Read the model definition and answer for the solid it produces. Units are mm, in the model's axes. A direction names the side the tool comes from. Coordinates: 2 decimals unless noted, no trailing zeros. Loops run counter-clockwise (first coordinate to the right, second up) from the corner with the lowest first, then second, coordinate; pieces in that order, holes last.
from build123d import *

# Parameters (mm, degrees)
F0_W      = 304.8
F0_H      = 304.8
F1_DEPTH  = 38.1
F2_W      = 228.6
F2_H      = 228.6
F3_DEPTH  = 38.1
F4_W      = 38.1
F4_H      = 38.1
F5_DEPTH  = 1143
F6_W      = 304.8
F6_H      = 304.8
F7_DEPTH  = 38.1
F8_W      = 228.6
F8_H      = 228.6
F9_DEPTH  = 38.1
F10_W     = 38.1
F10_H     = 38.1
F11_DEPTH = 342.9
F12_W     = 38.1
F12_H     = 38.1
F13_DEPTH = 342.9
F14_R     = 6.35
F16_DEPTH = 0.254
F15_R     = 6.35
F17_DEPTH = 0.254
F18_W     = 38.1
F18_H     = 38.1
F19_DEPTH = 304.8


with BuildPart() as f1:
    # F0 (on Top) → F1 (new body)
    with BuildSketch(Plane.XY):
        Rectangle(F0_W, F0_H)
    extrude(amount=-F1_DEPTH)

    # F2 (on face) → F3 (cut)
    with BuildSketch(Plane.XY):
        Rectangle(F2_W, F2_H)
    extrude(amount=-F3_DEPTH, mode=Mode.SUBTRACT)

    # F4 (on face) → F5 (join)
    with BuildSketch(Plane.XY):
        with Locations((-133.35, 133.35)):
            Rectangle(F4_W, F4_H)
        with Locations((133.35, 133.35)):
            Rectangle(F4_W, F4_H)
        with Locations((133.35, -133.35)):
            Rectangle(F4_W, F4_H)
        with Locations((-133.35, -133.35)):
            Rectangle(F4_W, F4_H)
    extrude(amount=F5_DEPTH)

    # F6 (on face) → F7 (join)
    with BuildSketch(Plane.XY.offset(1143)):
        Rectangle(F6_W, F6_H)
    extrude(amount=F7_DEPTH)

    # F8 (on face) → F9 (cut)
    with BuildSketch(Plane.XY.offset(1181.1)):
        Rectangle(F8_W, F8_H)
    extrude(amount=-F9_DEPTH, mode=Mode.SUBTRACT)

    # F10 (on face) → F11 (join)
    with BuildSketch(Plane(origin=(0, 0, 1143), x_dir=(1, 0, 0), z_dir=(0, 0, -1))):
        with Locations((133.35, 95.25)):
            Rectangle(F10_W, F10_H)
        with Locations((133.35, -95.25)):
            Rectangle(F10_W, F10_H)
    extrude(amount=F11_DEPTH)

    # F12 (on face) → F13 (join)
    with BuildSketch(Plane(origin=(0, 0, 1143), x_dir=(1, 0, 0), z_dir=(0, 0, -1))):
        with Locations((-133.35, -95.25)):
            Rectangle(F12_W, F12_H)
        with Locations((-133.35, 95.25)):
            Rectangle(F12_W, F12_H)
    extrude(amount=F13_DEPTH)

    # F14 (on face) → F16 (cut)
    with BuildSketch(Plane.YZ.offset(-114.3)):
        with Locations((95.25, 819.15)):
            Circle(F14_R)
        with Locations((-95.25, 819.15)):
            Circle(F14_R)
    extrude(amount=-F16_DEPTH, mode=Mode.SUBTRACT)

    # F15 (on face) → F17 (cut)
    with BuildSketch(Plane(origin=(114.3, 0, 0), x_dir=(0, -1, 0), z_dir=(-1, 0, 0))):
        with Locations((-95.25, 819.15)):
            Circle(F15_R)
        with Locations((95.25, 819.15)):
            Circle(F15_R)
    extrude(amount=-F17_DEPTH, mode=Mode.SUBTRACT)

    # F18 (on Front) → F19 (join, symmetric)
    with BuildSketch(Plane.XZ):
        with Locations((133.35, -19.05)):
            Rectangle(F18_W, F18_H)
        with Locations((-133.35, -19.05)):
            Rectangle(F18_W, F18_H)
    extrude(amount=F19_DEPTH, both=True)


solid = f1.part
Q1. Straight lines are drawn through the part: probe 1 along Y at (x, z) = (114.5, 819.15); probe 2 along Z at (x, y) = (-114.4, -95.25); probe 3 along Y at (x, z) = (125.5, 347). For each, find the intervals that lie inside material, in ascending order.
Findings below:
probe 1: y = -152.4 to -101.6, -88.9 to -76.2, 76.2 to 88.9, 101.6 to 152.4
probe 2: z = -38.1 to 0, 800.1 to 812.8, 825.5 to 1181.1
probe 3: y = -152.4 to -114.3, 114.3 to 152.4
Q2. Determine the mould class of faces 4 (the face through (-2, -114.3, -19)), 5 (the face through (-2, -140, -38.1)), 6 (the face through (133, -96, 800.1)), 7 (the face through (-134, 228, 0)) for opening direction Z: +Z half, -Z half, draft (parallel to the pull), parting line (faces both ways), or undercut.
Findings below:
face 4: draft
face 5: -Z half
face 6: undercut
face 7: +Z half
Q3. A cutting plane is placed at C-C (y = -179.5). Give the vertices of the cut face in (x, z), then the cut area to 3 significant figures.
Findings below:
outline: (-152.4, -38.1) - (-114.3, -38.1) - (-114.3, 0) - (-152.4, 0) - close; (114.3, -38.1) - (152.4, -38.1) - (152.4, 0) - (114.3, 0) - close
area: 2,900 mm2
Q4. Flat-ended cylindrical pins translate along their axes: pin 1 Ø4 at (x, y) = (-113, -207) entering from +Z; pin 2 Ø11.5 at (x, z) = (135, 226) entering from +Y. Find the tip coordinate at first contact, or state that the pin passes through.
Findings below:
pin 1: stops at z = 0
pin 2: stops at y = 152.4
Q5. A cutting plane is placed at A-A (y = 13.5). Give the vertices of the cut face in (x, z), then the cut area to 3 significant figures.
Findings below:
outline: (-152.4, -38.1) - (-114.3, -38.1) - (-114.3, 0) - (-152.4, 0) - close; (-152.4, 1143) - (-114.3, 1143) - (-114.3, 1181.1) - (-152.4, 1181.1) - close; (114.3, -38.1) - (152.4, -38.1) - (152.4, 0) - (114.3, 0) - close; (114.3, 1143) - (152.4, 1143) - (152.4, 1181.1) - (114.3, 1181.1) - close
area: 5,810 mm2
Q6. Which of the six approach directions +Z, -Z, +X, -X, +Y, -Y give full straight-line access (tool end or side, diameter ignored) to faces 1 (the face through (133, 230, 0)), 2 (the face through (114.3, 230, -19)), 3 (the face through (114.3, -228, -19))?
Findings below:
face 1: +Z, +X, -X, +Y
face 2: +Z, -Z, +Y
face 3: +Z, -Z, -Y
